from build123d import *

# Parameters (mm, degrees)
EXTRUDE_THIN1_DEPTH = 100
CUT_EXTRUDE1_DEPTH  = 1218
SKETCH4_R           = 10
CUT_EXTRUDE2_DEPTH  = 1285
FILLET1_R           = 35


with BuildPart() as part:
    # Sketch2 → Extrude-Thin1 (new, symmetric)
    with BuildSketch(Plane.XY):
        with BuildLine():
            Line((-500, 0), (-500, 80))
            ThreePointArc((-500, 80), (-494.142135624, 94.142135624), (-480, 100))
            Line((-480, 100), (480, 100))
            ThreePointArc((480, 100), (494.142135624, 94.142135624), (500, 80))
            Line((500, 80), (500, 0))
            Line((500, 0), (490, 0))
            Line((490, 0), (490, 80))
            ThreePointArc((490, 80), (487.071067812, 87.071067812), (480, 90))
            Line((480, 90), (-480, 90))
            ThreePointArc((-480, 90), (-487.071067812, 87.071067812), (-490, 80))
            Line((-490, 80), (-490, 0))
            Line((-490, 0), (-500, 0))
        make_face()
    extrude(amount=EXTRUDE_THIN1_DEPTH, both=True)

    # Sketch3 → Cut-Extrude1 (cut)
    with BuildSketch(Plane.ZY.offset(500)):
        Polygon((-100, 80), (-100, 0), (-50, 0), align=None)
    extrude(amount=-CUT_EXTRUDE1_DEPTH, mode=Mode.SUBTRACT)

    # Sketch4 → Cut-Extrude2 (cut)
    with BuildSketch(Plane.ZY.offset(500)):
        with Locations((60, 40)):
            Circle(SKETCH4_R)
    extrude(amount=-CUT_EXTRUDE2_DEPTH, mode=Mode.SUBTRACT)

    # Fillet1
    fillet1_edges = [part.edges().sort_by_distance(p)[0] for p in [
        (-495, 0, 100),
        (495, 0, 100),
    ]]
    fillet(fillet1_edges, radius=FILLET1_R)


solid = part.part
Here's how the part is built. I have some questions about the finished solid (model axes, mm). A direction names the side the tool comes from. Coordinates: 2 decimals unless noted, no trailing zeros. Write each loop counter-clockwise with the first axis right and the second up, starting at its lowest first coordinate (ties: lowest second). Pieces come first, ordered by that corner, then holes.
Item 1: On a 3-axis mill with a long thin cutter (end or side, diameter ignored), from which of +Z, -Z, +X, -X, +Y, -Y can I reach the whole of each face in a straight line? I mean faces 4 (the flat face through (490, 39, 1)), 5 (the flat face through (2, 94, 100)). Say none if no direction works.
Item 2: I want a section at B-B on y = 11. Write out the boundary of the cut face in (x, z) (3 decimals).
Item 3: If we mould it in two halves opening along Z, with no side actions, what happens to faces 1 (the flat face through (500, 41, 1)), 2 (the cylindrical face through (495, 34, 52)), 3 (the cylindrical face through (-495.07, 9.981, 89.475))? For each: +Z half, -Z half, draft (parallel to the pull), parting line (faces both ways), or undercut.
Item 4: If I drill on line 1 (X direction, y = 36, z = -15.5); line 2 (Y direction, x = 496, z = 60); line 3 (Y direction, x = -493, z = 60), over which ranges is the centre line in solid material (lowest first)?
Item 5: I want a section at C-C on x = -224. Write out the boundary of the cut face in (y, z).
Item 6: Will this pin go through, and if not, where does the flat tip stop? pin 1 (2 mm diameter, centred on x = -57, z = -41.5, fed in from -Y).
Item 7: I want a section at D-D on z = -71. Write out the boundary of the cut face in (x, y), and give its area (3 significant figures).
Item 8: I want a section at A-A on z = -16. Write out the boundary of the cut face in (x, y).
Findings below:
1. face 4: +Z, -Z, -Y
1. face 5: +Z, +X, -X, +Y, -Y
2. outline: (-500, -56.875) - (-490, -56.875) - (-490, 90.475) - (-500, 90.475) - close; (490, -56.875) - (500, -56.875) - (500, 90.475) - (490, 90.475) - close
3. face 1: draft
3. face 2: undercut
3. face 3: +Z half
4. line 1: x = -500 to -490, 490 to 500
4. line 2: y = 0 to 30, 50 to 92
4. line 3: y = 0 to 30, 50 to 95.2
5. outline: (90, -100) - (100, -100) - (100, 100) - (90, 100) - close
6. pin 1: stops at y = 90
7. outline: (-500, 33.6) - (-490, 33.6) - (-490, 80) arc R10 cw to (-480, 90) - (480, 90) arc R10 cw to (490, 80) - (490, 33.6) - (500, 33.6) - (500, 80) arc R20 ccw to (480, 100) - (-480, 100) arc R20 ccw to (-500, 80) - close
7. area: 11,000 mm2
8. outline: (-500, 0) - (-490, 0) - (-490, 80) arc R10 cw to (-480, 90) - (480, 90) arc R10 cw to (490, 80) - (490, 0) - (500, 0) - (500, 80) arc R20 ccw to (480, 100) - (-480, 100) arc R20 ccw to (-500, 80) - close
